Build history of the part. All positions in model axes, mm. A direction names the side the tool comes from. Round coordinates to 2 decimals unless told otherwise and drop trailing zeros. Write each loop counter-clockwise with the first axis right and the second up, starting at its lowest first coordinate (ties: lowest second). Pieces come first, ordered by that corner, then holes. Notation, with made-up numbers: M -30,53.25 L 14,53.25 A8 cw 14,68.25 Z; hole C 51,89 d7. An arc over 180 degrees is marked long. Write item = value, one per line. Start each with the question number.
Q1. Tool access for faces 4 (the flat face through (0.2, 1, 14)), 5 (the flat face through (0.2, -1, 1)), 6 (the flat face through (-0.2, 1, 14)): list every direction of +Z, -Z, +X, -X, +Y, -Y with a clear straight run to the whole face (end or side of a thin tool).
Q2. Band-saw the part on B-B on z = 4.5. Write the cut outline in (x, y), plus the area to 3 significant figures.
Q3. Band-saw the part on A-A on x = -0.95. Write the cut outline in (y, z).
Q4. Pull direction Z, two halves, no side cores. Call faces 1 (the flat face through (0, 0, 0)), 2 (the flat face through (-1.43, 0, 2.1)), 3 (the flat face through (-0.2, 1, 1)): released by +Z, released by -Z, zero draft, split by the parting line, or undercut.
Q5. Band-saw the part on C-C on x = 1.95. Write the cut outline in (y, z), plus the area to 3 significant figures.
Q6. Drop flat-ended pins along their axis: P1, Ø0.5, axis at x = -1, z = 16, coming from the -Y side; P2, Ø2, axis at x = -0.5, z = 9.5, coming from the -Y side; P3, Ø0.9, axis at y = -1, z = 16.5, coming from the -X side. Give the stop position or say it passes through.
Q7. Probe L1, parallel to Y at x = 0.85, z = 15.5; L2, parallel to Z at x = -0.1, y = -1. List the from-to ranges inside material, lowest first.
```python
from build123d import *

# Parameters (mm, degrees)
F3_DEPTH = 0.2
F4_COUNT = 4


# Not quite as in the source:
# - a feature names something its author has since deleted; it is built from what else it names


with BuildPart() as f1:
    # F0 (on Front) → F1 (revolve)
    with BuildSketch(Plane.XZ):
        with BuildLine():
            Line((0, 18.8888888889), (0, 0))
            Line((0, 0), (0.5451388889, 0))
            Line((0.5451388889, 0), (0.5451388889, 17.0138888889))
            ThreePointArc((0.5451388889, 17.0138888889), (0.53654676, 17.7085458509), (0.5107756304, 18.4027777778))
            ThreePointArc((0.5107756304, 18.4027777778), (0.3525605469, 18.7479364578), (0, 18.8888888889))
        make_face()
    revolve(axis=Axis((0, 0, 9.4444444444), (0, 0, 1)))

    # F2 (on Front) → F3 (join, symmetric)
    with BuildSketch(Plane.XZ):
        Polygon((0, 16.9097222222), (0, 0.1708931289), (2.3194444444, 0.0347222222), (2.3194444444, 1.6319444444), (0.4, 2.6461323114), (0.4, 13.75), (1.5972222222, 13.75), (1.5972222222, 13.8888888889), (1.2847222222, 14.375), (1.2847222222, 14.9652777778), (0.4, 14.9652777778), (0.4, 15.3125), (1.5972222222, 15.3125), (1.5972222222, 15.8333333333), (0.6493055556, 16.9097222222), align=None)
    extrude(amount=F3_DEPTH, both=True)

    # F4: F1 ×4 about axis
    f4_axis = Axis((0, 0, 0), (0, 0, 1))


with BuildPart() as f1_1:
    add(f1.part)
    for i in range(1, F4_COUNT):
        add(f1.part.rotate(f4_axis, i * 360 / F4_COUNT))


solid = f1_1.part
```
Conclusion:
q1.face_4 = +Z, -Z, +X, +Y
q1.face_5 = +Z, -Z, +X, -Y
q1.face_6 = +Z, -Z, -X, +Y
q2.outline = C 0,0 d1.09
q2.area = 0.934 mm^2
q3.outline = M -0.2,0.12 L 0.2,0.12 L 0.2,2.36 L -0.2,2.36 Z; M -0.2,13.75 L 0.2,13.75 L 0.2,14.97 L -0.2,14.97 Z; M -0.2,15.31 L 0.2,15.31 L 0.2,16.57 L -0.2,16.57 Z
q4.face_1 = released by -Z
q4.face_2 = undercut
q4.face_3 = zero draft
q5.outline = M -0.2,0.06 L 0.2,0.06 L 0.2,1.83 L -0.2,1.83 Z
q5.area = 0.708 mm^2
q6.P1 = -0.2
q6.P2 = -0.55
q6.P3 = -0.2
q7.L1 = -0.2 to 0.2
q7.L2 = 0.11 to 2.33, 13.75 to 14.97, 15.31 to 16.51
